Could you check a few things on this drawing? It's one solid part, dimensions in mm from its lowest x, y, z. Round coordinates to 2 decimals unless told otherwise and drop trailing zeros. Loops run counter-clockwise (first coordinate to the right, second up) from the corner with the lowest first, then second, coordinate; pieces in that order, holes last.
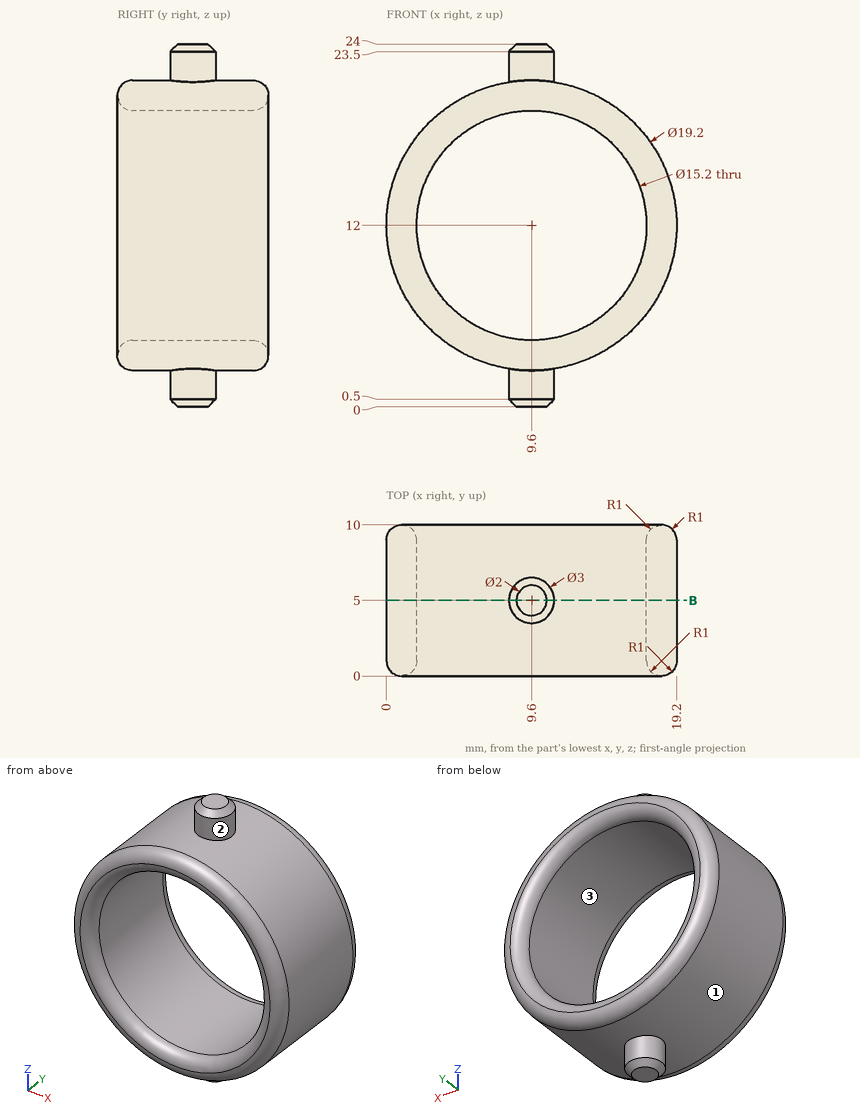
(1) We'd pull the mould along Z, two halves only. Please class the marked faces 1, 2 and 3: released by +Z, released by -Z, zero draft, split by the parting line, or undercut.
(2) Suppose I cut it at B-B (y = 5). Write out the boundary of the cut face in (x, z), then the cut area to 3 significant figures.
(3) If I drill on line 1 (X direction, y = 6, z = 12); line 2 (X direction, y = 5, z = 1.5); line 3 (Z direction, x = 16, y = 8.75) (1 decimal), over which ranges is the centre line in solid material (lowest first)?
(4) For pin 1 (5 mm diameter, centred on x = 2.5, y = 1.5, fed in from +Z); pin 2 (5 mm diameter, centred on y = 5, z = 17.5, fed in from +X); pin 3 (5 mm diameter, centred on x = 17, y = 8, fed in from +Z) (1 decimal), each with a flat end and sliding along its axis, tell me the tip position at first contact or that it passes through.
Check result:
1. face 1: split by the parting line
1. face 2: zero draft
1. face 3: undercut
2. outline: (8.1, 0.5) - (8.6, 0) - (10.6, 0) - (11.1, 0.5) - (11.1, 2.52) arc R9.6 ccw to (11.1, 21.48) - (11.1, 23.5) - (10.6, 24) - (8.6, 24) - (8.1, 23.5) - (8.1, 21.48) arc R9.6 ccw to (8.1, 2.52) - close; hole circle Ø15.2 at (9.6, 12)
2. area: 122 mm2
3. line 1: x = 0 to 2, 17.2 to 19.2
3. line 2: x = 8.1 to 11.1
3. line 3: z = 4.8 to 7.9, 16.1 to 19.2
4. pin 1: stops at z = 20.43
4. pin 2: stops at x = 18.72
4. pin 3: stops at z = 20.3
